Input: dimensioned drawing with shaded views. Units: mm. Origin: part minimum x, y, z. A direction names the side the tool comes from. Round coordinates to 2 decimals unless told otherwise and drop trailing zeros. Order: outer loops, then holes, each group sorted by start corner. A loop starts at its lowest first (then second) coordinate and runs counter-clockwise, first axis right, second up. Notation, with made-up numbers: M -34.75,41.5 L -29.75,41.5 A18 cw -29.75,55.5 Z; hole C 28,48 d4. An arc over 180 degrees is marked long. Use one line per item in the form item = value. Start each with the question number.
Q1. Section B-B (x = 3.75). Return the cut outline in (y, z) (1 decimal).
Q2. Section A-A (z = 132.5). Return the cut outline in (x, y), plus the area to 3 significant figures.
Q3. Pull-direction query (Y, two-part tool) for the marked faces 3, 4 and 5; classes: pulls with the +Y half, pulls with the -Y half, needs draft (parallel to the pull), parting line crosses it, or undercut.
Q4. Reachability of the marked faces 1 and 2 from +Z, -Z, +X, -X, +Y, -Y: full face, straight path, thin tool, end or side. Return the list, or none.
Q5. Material intervals for probe 1 along Y at (x, z) = (10.5, 63.5), sorted ascending.
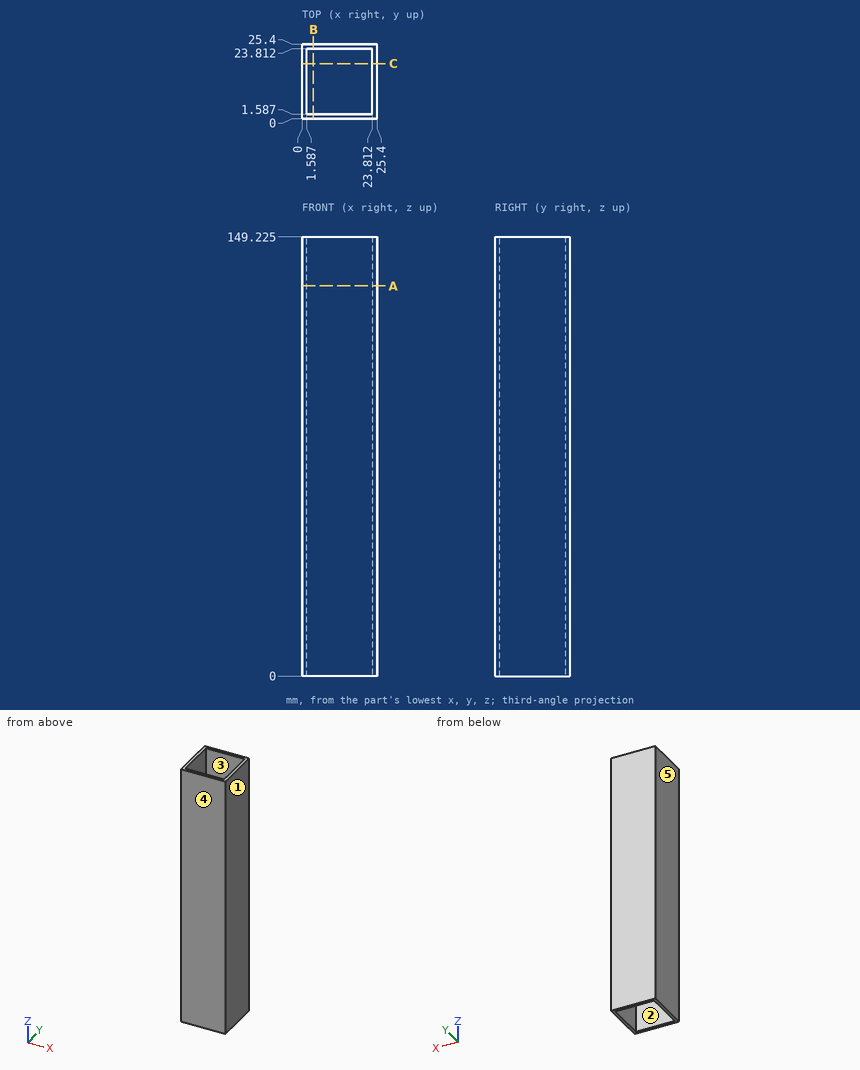
Results list:
q1.outline = M 0,0 L 1.6,0 L 1.6,149.2 L 0,149.2 Z; M 23.8,0 L 25.4,0 L 25.4,149.2 L 23.8,149.2 Z
q2.outline = M 0,0 L 25.4,0 L 25.4,25.4 L 0,25.4 Z; hole M 1.59,1.59 L 23.81,1.59 L 23.81,23.81 L 1.59,23.81 Z
q2.area = 151 mm2
q3.face_3 = undercut
q3.face_4 = pulls with the -Y half
q3.face_5 = needs draft
q4.face_1 = +Z, -Z, +X, +Y, -Y
q4.face_2 = +Z, -Z
q5.probe_1 = 0 to 1.59, 23.81 to 25.4
